Read the model definition and answer for the solid it produces. Units are mm, in the model's axes. Face numbers are marked on the shaded views. A direction names the side the tool comes from. Coordinates: 2 decimals unless noted, no trailing zeros. Write each loop counter-clockwise with the first axis right and the second up, starting at its lowest first coordinate (ties: lowest second). Pieces come first, ordered by that corner, then holes. Notation, with made-up numbers: (18, 82.25) -> (43, 82.25) arc R18 ccw to (43, 106.25) -> close; hole circle Ø2 at (52.5, -6.75). An arc over 180 degrees is marked (long way). Answer in a Markdown table with one row per item. Add a question column.
Item 1: Straight lines are drawn through the part: line 1 (X direction, y = 0, z = 28); line 2 (Y direction, x = 0, z = 21.25); line 3 (Z direction, x = -51, y = 15.5). For each, find the intervals that lie inside material, in ascending order. Write a range as from..to.
Item 2: For a pull along Z with two mould halves and no side action, classify the marked faces 4, 5, 6 and 7 as +Z half, -Z half, draft (parallel to the pull), parting line (faces both ways), or undercut.
Item 3: Section C-C on y = 32.75 is taken. Write down the section's boundary in (x, z), then the cut area to 3 significant figures.
Item 4: Section D-D on x = 0 is taken. Count the separate pieces of the cut face and the enclosed holes in it, then the cut area to 3 significant figures.
Item 5: Which of the six approach directions +Z, -Z, +X, -X, +Y, -Y give full straight-line access (tool end or side, diameter ignored) to the marked faces 1, 2 and 3?
Item 6: Section B-B on z = 7 is taken. Write down the section's boundary in (x, y).
Item 7: Given pin 1 Ø1.5 at (x, y) = (9.5, -3.5) entering from -Z; pin 2 Ø13 at (x, z) = (-36, 3) entering from -Y; pin 3 Ø4 at (x, y) = (7, 0) entering from -Z, each flat-ended and moving along its own axis, determine where each tip first touches the part or whether it passes through.
Item 8: Section A-A on x = -36.5 is taken. Write down the section's boundary in (y, z).
```python
from build123d import *
from build123d.topology import SkipClean

# Parameters (mm, degrees)
S_CYL1_R        = 19
BOSS_1_DEPTH    = 7
BOSS_2_DEPTH    = 2.1
S_BOX3_W        = 28.2
S_BOX3_H        = 10
BOSS_3_DEPTH    = 1.5
S_BOX4_W        = 37.6
S_BOX4_H        = 47
BOSS_4_DEPTH    = 14.2
S_BOX5_W        = 36.1
S_BOX5_H        = 3
BOSS_5_DEPTH    = 31.8
S_BOX6_W        = 36.1
S_BOX6_H        = 3
BOSS_6_DEPTH    = 31.8
S_BOX7_W        = 36.1
S_BOX7_H        = 52.4
BOSS_7_DEPTH    = 3
S_BOX8_W        = 36.1
S_BOX8_H        = 52.4
BOSS_8_DEPTH    = 3
S_BOX9_W        = 4.6
S_BOX9_H        = 52.4
BOSS_9_DEPTH    = 31.8
S_HOLE10_R      = 10.5
HOLE_10_DEPTH   = 4.8
S_CUT11_W       = 4.75
S_CUT11_H       = 19.5
POCKET_11_DEPTH = 19.4
S_CUT12_W       = 4.75
S_CUT12_H       = 8.8
POCKET_12_DEPTH = 16.4
S_CUT13_W       = 4.75
S_CUT13_H       = 11
POCKET_13_DEPTH = 7
S_CUT14_W       = 2.9
S_CUT14_H       = 20
POCKET_14_DEPTH = 16.4
S_HOLE15_R      = 1.1
HOLE_15_DEPTH   = 4.8
S_HOLE16_R      = 2.3
HOLE_16_DEPTH   = 1.7
S_HOLE17_R      = 1.1
HOLE_17_DEPTH   = 4.8
S_HOLE18_R      = 2.3
HOLE_18_DEPTH   = 1.7
S_HOLE19_R      = 1.1
HOLE_19_DEPTH   = 4.8
S_HOLE20_R      = 2.3
HOLE_20_DEPTH   = 1.7
CUT_21_DEPTH    = 6.1
S_HOLE22_R      = 3.5
HOLE_22_DEPTH   = 10.6
S_HOLE23_R      = 1.7
HOLE_23_DEPTH   = 10.6
S_HOLE24_R      = 1.7
HOLE_24_DEPTH   = 10.6
S_HOLE25_R      = 1.7
HOLE_25_DEPTH   = 10.6
S_HOLE26_R      = 1.7
HOLE_26_DEPTH   = 10.6
S_HOLE27_R      = 3.2
HOLE_27_DEPTH   = 7.6
S_HOLE28_R      = 3.2
HOLE_28_DEPTH   = 7.6
S_HOLE29_R      = 3.2
HOLE_29_DEPTH   = 7.6
S_HOLE30_R      = 3.2
HOLE_30_DEPTH   = 7.6


with BuildPart() as part:
    # S_cyl1 → Boss_1 (new body)
    with BuildSketch(Plane.XY.offset(23)):
        Circle(S_CYL1_R)
    extrude(amount=BOSS_1_DEPTH)

    # S_prism2 → Boss_2 (add)
    with SkipClean():  # the faces are left unmerged after this step: merging them gives an invalid solid
        with BuildSketch(Plane.XY.offset(21)):
            with BuildLine():
                Line((-15.491933385, 11), (15.491933385, 11))
                ThreePointArc((15.491933385, 11), (19, 0), (15.491933385, -11))
                Line((15.491933385, -11), (-15.491933385, -11))
                ThreePointArc((-15.491933385, -11), (-19, 0), (-15.491933385, 11))
            make_face()
        extrude(amount=BOSS_2_DEPTH)

    # S_box3 → Boss_3 (add)
    with SkipClean():  # the faces are left unmerged after this step: merging them gives an invalid solid
        with BuildSketch(Plane.XY.offset(19.6)):
            with Locations((-0.1, 0)):
                Rectangle(S_BOX3_W, S_BOX3_H)
        extrude(amount=BOSS_3_DEPTH)

    # S_box4 → Boss_4 (add)
    with SkipClean():  # the faces are left unmerged after this step: merging them gives an invalid solid
        with BuildSketch(Plane.XY.offset(15.8)):
            with Locations((-35.2, 11.5)):
                Rectangle(S_BOX4_W, S_BOX4_H)
        extrude(amount=BOSS_4_DEPTH)

    # S_box6 → Boss_6 (add)
    with SkipClean():  # the faces are left unmerged after this step: merging them gives an invalid solid
        with BuildSketch(Plane.XY.offset(-15.9)):
            with Locations((-36.85, -12.2)):
                Rectangle(S_BOX6_W, S_BOX6_H)
        extrude(amount=BOSS_6_DEPTH)



with BuildPart() as body_2:
    # S_box5 → Boss_5 (new body)
    with BuildSketch(Plane.XY.offset(-15.9)):
        with Locations((-36.85, 37.2)):
            Rectangle(S_BOX5_W, S_BOX5_H)
    extrude(amount=BOSS_5_DEPTH)


with BuildPart() as part_1:
    with SkipClean():  # the faces are left unmerged after this step: merging them gives an invalid solid
        add(part.part)

        add(body_2.part)  # Boss_7 merges body 2
        # S_box7 → Boss_7 (add)
        with BuildSketch(Plane.XY.offset(-15.9)):
            with Locations((-36.85, 12.5)):
                Rectangle(S_BOX7_W, S_BOX7_H)
        extrude(amount=BOSS_7_DEPTH)

    # S_box8 → Boss_8 (add)
    with SkipClean():  # the faces are left unmerged after this step: merging them gives an invalid solid
        with BuildSketch(Plane.XY.offset(12.9)):
            with Locations((-36.85, 12.5)):
                Rectangle(S_BOX8_W, S_BOX8_H)
        extrude(amount=BOSS_8_DEPTH)

    # S_box9 → Boss_9 (add)
    with SkipClean():  # the faces are left unmerged after this step: merging them gives an invalid solid
        with BuildSketch(Plane.XY.offset(-15.9)):
            with Locations((-52.6, 12.5)):
                Rectangle(S_BOX9_W, S_BOX9_H)
        extrude(amount=BOSS_9_DEPTH)

    # S_hole10 → Hole_10 (cut)
    with SkipClean():  # the faces are left unmerged after this step: merging them gives an invalid solid
        with BuildSketch(Plane(origin=(-55, 0, 0), x_dir=(0, 0, -1), z_dir=(1, 0, 0))):
            with Locations(Location((0, 0, 0), (0, 0, 180))):
                Circle(S_HOLE10_R)
        extrude(amount=HOLE_10_DEPTH, mode=Mode.SUBTRACT)

    # S_cut11 → Pocket_11 (cut)
    with SkipClean():  # the faces are left unmerged after this step: merging them gives an invalid solid
        with BuildSketch(Plane.XY.offset(-9.7)):
            with Locations((-52.625, 20.65)):
                Rectangle(S_CUT11_W, S_CUT11_H)
        extrude(amount=POCKET_11_DEPTH, mode=Mode.SUBTRACT)

    # S_cut12 → Pocket_12 (cut)
    with SkipClean():  # the faces are left unmerged after this step: merging them gives an invalid solid
        with BuildSketch(Plane.XY.offset(-8.2)):
            with Locations((-52.625, 34.8)):
                Rectangle(S_CUT12_W, S_CUT12_H)
        extrude(amount=POCKET_12_DEPTH, mode=Mode.SUBTRACT)

    # S_cut13 → Pocket_13 (cut)
    with SkipClean():  # the faces are left unmerged after this step: merging them gives an invalid solid
        with BuildSketch(Plane.XY.offset(-3.5)):
            with Locations((-52.625, 5.5)):
                Rectangle(S_CUT13_W, S_CUT13_H)
        extrude(amount=POCKET_13_DEPTH, mode=Mode.SUBTRACT)

    # S_cut14 → Pocket_14 (cut)
    with SkipClean():  # the faces are left unmerged after this step: merging them gives an invalid solid
        with BuildSketch(Plane.XY.offset(-16.4)):
            with Locations((-53.65, 0)):
                Rectangle(S_CUT14_W, S_CUT14_H)
        extrude(amount=POCKET_14_DEPTH, mode=Mode.SUBTRACT)

    # S_hole15 → Hole_15 (cut)
    with SkipClean():  # the faces are left unmerged after this step: merging them gives an invalid solid
        with BuildSketch(Plane(origin=(-55, 0, 0), x_dir=(0, 0, -1), z_dir=(1, 0, 0))):
            with Locations(Location((-10.25, 8.3, 0), (0, 0, 180))):
                Circle(S_HOLE15_R)
        extrude(amount=HOLE_15_DEPTH, mode=Mode.SUBTRACT)

    # S_hole16 → Hole_16 (cut)
    with SkipClean():  # the faces are left unmerged after this step: merging them gives an invalid solid
        with BuildSketch(Plane(origin=(-55, 0, 0), x_dir=(0, 0, -1), z_dir=(1, 0, 0))):
            with Locations((-10.25, 8.3)):
                Circle(S_HOLE16_R)
        extrude(amount=HOLE_16_DEPTH, mode=Mode.SUBTRACT)

    # S_hole17 → Hole_17 (cut)
    with SkipClean():  # the faces are left unmerged after this step: merging them gives an invalid solid
        with BuildSketch(Plane(origin=(-55, 0, 0), x_dir=(0, 0, -1), z_dir=(1, 0, 0))):
            with Locations(Location((10.25, 32.75, 0), (0, 0, 180))):
                Circle(S_HOLE17_R)
        extrude(amount=HOLE_17_DEPTH, mode=Mode.SUBTRACT)

    # S_hole18 → Hole_18 (cut)
    with SkipClean():  # the faces are left unmerged after this step: merging them gives an invalid solid
        with BuildSketch(Plane(origin=(-55, 0, 0), x_dir=(0, 0, -1), z_dir=(1, 0, 0))):
            with Locations((10.25, 32.75)):
                Circle(S_HOLE18_R)
        extrude(amount=HOLE_18_DEPTH, mode=Mode.SUBTRACT)

    # S_hole19 → Hole_19 (cut)
    with SkipClean():  # the faces are left unmerged after this step: merging them gives an invalid solid
        with BuildSketch(Plane(origin=(-55, 0, 0), x_dir=(0, 0, -1), z_dir=(1, 0, 0))):
            with Locations(Location((-10.25, 32.75, 0), (0, 0, 180))):
                Circle(S_HOLE19_R)
        extrude(amount=HOLE_19_DEPTH, mode=Mode.SUBTRACT)

    # S_hole20 → Hole_20 (cut)
    with SkipClean():  # the faces are left unmerged after this step: merging them gives an invalid solid
        with BuildSketch(Plane(origin=(-55, 0, 0), x_dir=(0, 0, -1), z_dir=(1, 0, 0))):
            with Locations((-10.25, 32.75)):
                Circle(S_HOLE20_R)
        extrude(amount=HOLE_20_DEPTH, mode=Mode.SUBTRACT)

    # S_pcut21 → Cut_21 (cut)
    with BuildSketch(Plane.XY.offset(20.9)):
        with BuildLine():
            Line((-9.201642631, -17.30577282), (-7.182914911, -13.509098171))
            ThreePointArc((-7.182914911, -13.509098171), (13.316442148, -7.53408047), (7.880082546, 13.114659701))
            Line((7.880082546, 13.114659701), (10.094746268, 16.800479094))
            ThreePointArc((10.094746268, 16.800479094), (17.05897164, -9.651501778), (-9.201642631, -17.30577282))
        make_face()
    extrude(amount=CUT_21_DEPTH, mode=Mode.SUBTRACT)

    # S_hole22 → Hole_22 (cut)
    with BuildSketch(Plane.XY.offset(19.5)):
        Circle(S_HOLE22_R)
    extrude(amount=HOLE_22_DEPTH, mode=Mode.SUBTRACT)

    # S_hole23 → Hole_23 (cut)
    with BuildSketch(Plane.XY.offset(19.5)):
        with Locations((7, 0)):
            Circle(S_HOLE23_R)
    extrude(amount=HOLE_23_DEPTH, mode=Mode.SUBTRACT)

    # S_hole24 → Hole_24 (cut)
    with BuildSketch(Plane.XY.offset(19.5)):
        with Locations(Location((0, -7, 0), (0, 0, 180))):
            Circle(S_HOLE24_R)
    extrude(amount=HOLE_24_DEPTH, mode=Mode.SUBTRACT)

    # S_hole25 → Hole_25 (cut)
    with BuildSketch(Plane.XY.offset(19.5)):
        with Locations((-7, 0)):
            Circle(S_HOLE25_R)
    extrude(amount=HOLE_25_DEPTH, mode=Mode.SUBTRACT)

    # S_hole26 → Hole_26 (cut)
    with BuildSketch(Plane.XY.offset(19.5)):
        with Locations(Location((0, 7, 0), (0, 0, 180))):
            Circle(S_HOLE26_R)
    extrude(amount=HOLE_26_DEPTH, mode=Mode.SUBTRACT)

    # S_hole27 → Hole_27 (cut)
    with BuildSketch(Plane.XY.offset(19.4)):
        with Locations(Location((7, 0, 0), (0, 0, 180))):
            Circle(S_HOLE27_R)
    extrude(amount=HOLE_27_DEPTH, mode=Mode.SUBTRACT)

    # S_hole28 → Hole_28 (cut)
    with BuildSketch(Plane.XY.offset(19.4)):
        with Locations(Location((0, -7, 0), (0, 0, 141.317812547))):
            Circle(S_HOLE28_R)
    extrude(amount=HOLE_28_DEPTH, mode=Mode.SUBTRACT)

    # S_hole29 → Hole_29 (cut)
    with BuildSketch(Plane.XY.offset(19.4)):
        with Locations(Location((-7, 0, 0), (0, 0, 180))):
            Circle(S_HOLE29_R)
    extrude(amount=HOLE_29_DEPTH, mode=Mode.SUBTRACT)

    # S_hole30 → Hole_30 (cut)
    with BuildSketch(Plane.XY.offset(19.4)):
        with Locations(Location((0, 7, 0), (0, 0, 218.682187453))):
            Circle(S_HOLE30_R)
    extrude(amount=HOLE_30_DEPTH, mode=Mode.SUBTRACT)


solid = part_1.part
```
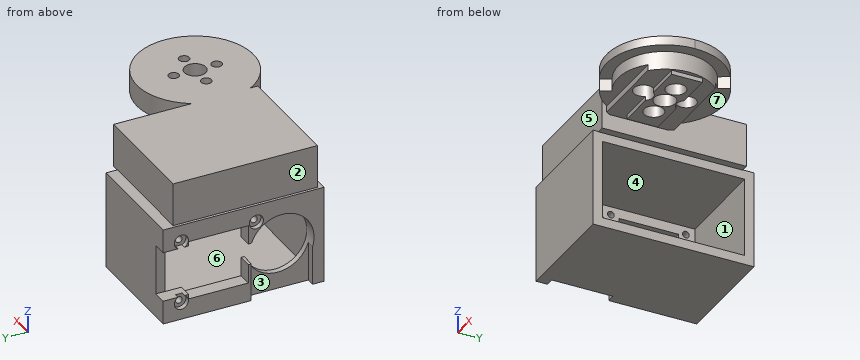
Results below:
| question | item | result |
|---|---|---|
| 1 | line 1 | x = -54..-8.7, -5.3..-3.5, 3.5..5.3, 8.7..19 |
| 1 | line 2 | y = -11..-10.2, -3.8..-3.5, 3.5..3.8, 10.2..11 |
| 1 | line 3 | z = -15.9..-9.7, 9.7..30 |
| 2 | face 4 | undercut |
| 2 | face 5 | draft |
| 2 | face 6 | undercut |
| 2 | face 7 | -Z half |
| 3 | outline | (-54.9, -15.9) -> (-18.8, -15.9) -> (-18.8, -12.9) -> (-50.3, -12.9) -> (-50.3, -11.35) -> (-53.3, -11.35) -> (-53.3, -12.55) -> (-54.9, -12.55) -> close; (-54.9, 12.55) -> (-53.3, 12.55) -> (-53.3, 11.35) -> (-50.3, 11.35) -> (-50.3, 12.9) -> (-18.8, 12.9) -> (-18.8, 15.8) -> (-16.4, 15.8) -> (-16.4, 30) -> (-54, 30) -> (-54, 15.9) -> (-54.9, 15.9) -> close; (-53.3, -9.15) -> (-50.3, -9.15) -> (-50.3, -8.2) -> (-53.3, -8.2) -> close; (-53.3, 8.2) -> (-50.3, 8.2) -> (-50.3, 9.15) -> (-53.3, 9.15) -> close |
| 3 | area | 763 mm2 |
| 4 | separate pieces | 4 |
| 4 | enclosed holes | 0 |
| 4 | area | 136 mm2 |
| 5 | face 1 | +X |
| 5 | face 2 | +Z, -X, +Y, -Y |
| 5 | face 3 | -Z, -X |
| 6 | outline | (-54.9, -13.7) -> (-18.8, -13.7) -> (-18.8, -10.7) -> (-50.3, -10.7) -> (-50.3, -7.83) -> (-54.9, -7.83) -> close; (-54.9, 7.83) -> (-50.3, 7.83) -> (-50.3, 10.9) -> (-54.9, 10.9) -> close; (-50.25, 35.7) -> (-18.8, 35.7) -> (-18.8, 38.7) -> (-50.25, 38.7) -> close |
| 7 | pin 1 | stops at z = 19.6 |
| 7 | pin 2 | stops at y = -13.7 |
| 7 | pin 3 | stops at z = 27 |
| 8 | outline | (-13.7, -15.9) -> (38.7, -15.9) -> (38.7, 15.9) -> (35, 15.9) -> (35, 30) -> (-12, 30) -> (-12, 15.9) -> (-13.7, 15.9) -> close; hole (-10.7, -12.9) -> (35.7, -12.9) -> (35.7, 12.9) -> (-10.7, 12.9) -> close |
